Geometry check sheet. Reference: the model listing, model coordinates, mm. A direction names the side the tool comes from. Coordinates: 2 decimals unless noted, no trailing zeros. Write each loop counter-clockwise with the first axis right and the second up, starting at its lowest first coordinate (ties: lowest second). Pieces come first, ordered by that corner, then holes. Notation, with made-up numbers: M 41.25,45 L 65.25,45 A21 cw 65.25,70 Z; hole C 5,85.25 d1. An arc over 180 degrees is marked long. Write each question's results on one line, items separated by ' | '.
```python
from build123d import *

# Parameters (mm, degrees)
F0_W     = 280
F0_H     = 110
F1_DEPTH = 2
F2_R     = 3.5
F2_R_2   = 3.15
F3_DEPTH = 25
F4_R     = 2
F4_R_2   = 1.75
F5_DEPTH = 25
F6_W     = 27.2
F6_H     = 46.7
F7_DEPTH = 1


with BuildPart() as f1:
    # F0 (on Top) → F1 (new body)
    with BuildSketch(Plane.XY):
        with Locations((-90.244181, 21.321014)):
            Rectangle(F0_W, F0_H)
    extrude(amount=F1_DEPTH)

    # F2 (on face) → F3 (cut)
    with BuildSketch(Plane.XY.offset(2)):
        with Locations((-174.041525, 37.321014)):
            Circle(F2_R)
        with Locations((-150.041525, 37.321014)):
            Circle(F2_R)
        with Locations((-126.041525, 37.321014)):
            Circle(F2_R)
        with Locations((-102.041525, 37.321014)):
            Circle(F2_R)
        with Locations((-26.333425, 37.321014)):
            Circle(F2_R)
        with Locations((-13.643486, 3.923428)):
            Circle(F2_R_2)
        with Locations((-38.643486, 3.923428)):
            Circle(F2_R_2)
    extrude(amount=-F3_DEPTH, mode=Mode.SUBTRACT)

    # F4 (on face) → F5 (cut)
    with BuildSketch(Plane(origin=(0, 0, 0), x_dir=(1, 0, 0), z_dir=(0, 0, -1))):
        with Locations((6.512116, -36.321014)):
            Circle(F4_R)
        with Locations((-20.487884, -36.321014)):
            Circle(F4_R)
        with Locations((-47.487884, -36.321014)):
            Circle(F4_R)
        with Locations((-74.487884, -36.321014)):
            Circle(F4_R)
        with Locations((-221.244181, 24.678986)):
            Circle(F4_R_2)
        with Locations((-221.244181, -67.321014)):
            Circle(F4_R_2)
        with Locations((40.755819, 24.678986)):
            Circle(F4_R_2)
        with Locations((40.755819, -67.321014)):
            Circle(F4_R_2)
        with Locations((-167.244181, 24.678986)):
            Circle(F4_R_2)
        with Locations((-167.244181, -67.321014)):
            Circle(F4_R_2)
        with Locations((-113.244181, 24.678986)):
            Circle(F4_R_2)
        with Locations((-113.244181, -67.321014)):
            Circle(F4_R_2)
        with Locations((-59.244181, 24.678986)):
            Circle(F4_R_2)
        with Locations((-59.244181, -67.321014)):
            Circle(F4_R_2)
        with Locations((-5.244181, 24.678986)):
            Circle(F4_R_2)
        with Locations((-5.244181, -67.321014)):
            Circle(F4_R_2)
        with Locations((-221.244181, -17.321014)):
            Circle(F4_R_2)
        with Locations((40.755819, -17.321014)):
            Circle(F4_R_2)
    extrude(amount=-F5_DEPTH, mode=Mode.SUBTRACT)

    # F6 (on face) → F7 (cut)
    with BuildSketch(Plane.XY.offset(2)):
        with Locations((-187.032314, 15.971014)):
            Rectangle(F6_W, F6_H)
    extrude(amount=-F7_DEPTH, mode=Mode.SUBTRACT)


solid = f1.part
```
Q1. Access from +Z, -Z, +X, -X, +Y, -Y to the whole of each face (thin tool, end or side, straight path). Record for faces 1 (the cylindrical face through (-172.16, 40.27, 1.01)), 2 (the flat face through (-187, 16, 1)).
Geometry check:
face 1: +Z, -Z | face 2: +Z
Q2. Sectioned sample at A-A on y = 28.5. Record the cut outline in (x, z).
Geometry check:
outline: M -230.24,0 L 49.76,0 L 49.76,2 L -173.43,2 L -173.43,1 L -200.63,1 L -200.63,2 L -230.24,2 Z
Q3. Sectioned sample at B-B on z = 1.35. Give the number of separate pieces and of enclosed holes in the cut face, and give its area (3 significant figures).
Geometry check:
separate pieces: 1 | enclosed holes: 25 | area: 29,100 mm2
Q4. Scan lines: probe 1 along Y at (x, z) = (-26, 0.55); probe 2 along X at (y, z) = (2, 1.15); probe 3 along Y at (x, z) = (-148, 0.4). Record each from-to range of solid material in increasing order.
Geometry check:
probe 1: y = -33.68 to 33.84, 40.81 to 76.32 | probe 2: x = -230.24 to -200.63, -173.43 to -41.14, -36.15 to -16.14, -11.15 to 49.76 | probe 3: y = -33.68 to 34.48, 40.16 to 76.32
Q5. Mould release check, pull along Y, two halves, no side actions. Record for faces 3 (the cylindrical face through (-104.62, 39.69, 1.01)), 4 (the flat face through (-92, 22, 0)), 5 (the cylindrical face through (-35.64, 4.87, 1.01)): pulls with the +Y half, pulls with the -Y half, needs draft (parallel to the pull), parting line crosses it, or undercut.
Geometry check:
face 3: undercut | face 4: needs draft | face 5: undercut
Q6. Depth check by flat-ended pin: P1, Ø5.5, axis at x = -221.24, y = -24.68, coming from the -Z side; P2, Ø3, axis at x = 40.76, y = 17.32, coming from the +Z side. Enter the tip coordinate at first touch or a pass-through.
Geometry check:
P1: stops at z = 0 | P2: passes through
